Here's how the part is built. I have some questions about the finished solid (model axes, mm). A direction names the side the tool comes from. Give positions to 0.01 mm unless a question says otherwise; leave off trailing zeros. Write each loop counter-clockwise with the first axis right and the second up, starting at its lowest first coordinate (ties: lowest second). Pieces come first, ordered by that corner, then holes. Notation, with made-up numbers: (-24.75, 84.25) -> (-9.75, 84.25) arc R23 cw to (-9.75, 98.25) -> close; hole circle Ø5 at (28, 51). An arc over 180 degrees is marked (long way). Put each result on its own line as item: value. Start each with the question number.
from build123d import *

# Parameters (mm, degrees)
BOSS_EXTRUDE1_DEPTH = 20
SKETCH2_R           = 35
SKETCH2_R_2         = 20
BOSS_EXTRUDE2_DEPTH = 30
FILLET1_R           = 2
FILLET2_R           = 2


with BuildPart() as part:
    # Sketch1 → Revolve-Thin1 (revolve)
    with BuildSketch(Plane.XY, mode=Mode.PRIVATE) as revolve_thin1_sk:
        with BuildLine():
            Line((56.568542495, 20), (80, 20))
            ThreePointArc((80, 20), (81.025996139, 15.83772234), (84.898979486, 14))
            Line((84.898979486, 14), (150, 14))
            Line((150, 14), (150, 0))
            Line((150, 0), (140, 0))
            Line((140, 0), (140, 4))
            Line((140, 4), (84.898979486, 4))
            ThreePointArc((84.898979486, 4), (78.190775553, 5.583592135), (72.898979486, 10))
            Line((72.898979486, 10), (56.568542495, 10))
            Line((56.568542495, 10), (56.568542495, 20))
        make_face()
    revolve(revolve_thin1_sk.sketch.rotate(Axis((-93.302775415, 0, 0), (1, 0, 0)), 90), axis=Axis((-93.302775415, 0, 0), (1, 0, 0)))

    # Sketch1<4> → Boss-Extrude1 (add, symmetric)
    with BuildSketch(Plane.XY):
        with BuildLine():
            Line((0, 60), (-21.3, 60))
            Line((-21.3, 60), (-21.3, 40))
            Line((-21.3, 40), (0, 40))
            ThreePointArc((0, 40), (40, 0), (0, -40))
            Line((0, -40), (-21.3, -40))
            Line((-21.3, -40), (-21.3, -60))
            Line((-21.3, -60), (0, -60))
            ThreePointArc((0, -60), (60, 0), (0, 60))
        make_face()
    extrude(amount=BOSS_EXTRUDE1_DEPTH, both=True)

    # Sketch2 → Boss-Extrude2 (add)
    with BuildSketch(Plane(origin=(0, 40, 0), x_dir=(1, 0, 0), z_dir=(0, 1, 0))):
        with Locations(Location((-50, 0, 0), (0, 0, 34.849904579))):
            Circle(SKETCH2_R)
        with Locations(Location((-50, 0, 0), (0, 0, 270))):
            Circle(SKETCH2_R_2, mode=Mode.SUBTRACT)
    boss_extrude2 = extrude(amount=BOSS_EXTRUDE2_DEPTH)

    # Fillet1
    # the kernel refuses this fillet: 2 mm, written as the material it adds along each edge
    with BuildSketch(Plane(origin=(-50, 60, 0), x_dir=(0.7309132797972386, 0, -0.682470349111259), z_dir=(-0.682470349111259, 0, -0.7309132797972386))) as fillet1_piece_1_section:
        with BuildLine():
            CenterArc((35 + FILLET1_R, -FILLET1_R), FILLET1_R, 90, 90)
            Line((35, -FILLET1_R), (35, 0))
            Line((35, 0), (35 + FILLET1_R, 0))
        make_face()
    fillet1_piece_1 = revolve(axis=Axis((-50, 60, 0), (0, -1, 0)), revolution_arc=86.073975491, mode=Mode.PRIVATE)
    fillet1_piece_1 = split(fillet1_piece_1, bisect_by=Plane(origin=(-14.43905365, 60.56094635, -20), z_dir=(0, 0, 1)), keep=Keep.TOP, mode=Mode.PRIVATE)
    fillet1_piece_1 = split(fillet1_piece_1, bisect_by=Plane(origin=(-14.43905365, 60.56094635, 20), z_dir=(0, 0, -1)), keep=Keep.TOP, mode=Mode.PRIVATE)
    add(fillet1_piece_1)

    # Mirror3: Boss-Extrude2 across plane
    add(boss_extrude2.mirror(Plane.ZX))

    # Fillet2
    # the kernel refuses this fillet: 2 mm, written as the material it adds along each edge
    with BuildSketch(Plane(origin=(-50, -60, 0), x_dir=(0.7309132797966846, 0, 0.6824703491118522), z_dir=(-0.6824703491118522, 0, 0.7309132797966846))) as fillet2_piece_1_section:
        with BuildLine():
            CenterArc((35 + FILLET2_R, -FILLET2_R), FILLET2_R, 90, 90)
            Line((35, -FILLET2_R), (35, 0))
            Line((35, 0), (35 + FILLET2_R, 0))
        make_face()
    fillet2_piece_1 = revolve(axis=Axis((-50, -60, 0), (0, 1, 0)), revolution_arc=86.073975491, mode=Mode.PRIVATE)
    fillet2_piece_1 = split(fillet2_piece_1, bisect_by=Plane(origin=(-14.439053646, -60.560946354, -20), z_dir=(0, 0, 1)), keep=Keep.TOP, mode=Mode.PRIVATE)
    fillet2_piece_1 = split(fillet2_piece_1, bisect_by=Plane(origin=(-14.439053646, -60.560946354, 20), z_dir=(0, 0, -1)), keep=Keep.TOP, mode=Mode.PRIVATE)
    add(fillet2_piece_1)


solid = part.part
1) I'm going to push flat-ended pins straight in: pin 1 Ø5 at (x, z) = (28, -14) entering from +Y; pin 2 Ø9 at (y, z) = (0, 0) entering from -X; pin 3 Ø1 at (y, z) = (37.5, 3.5) entering from +X. Where does each tip first touch, or does it pass through?
2) I want a section at B-B, the plane z = 0. State how many separate pieces and enclosed holes the cut face has, and give its area (3 significant figures).
3) I want a section at A-A, the plane x = -50. Write out the boundary of the cut face in (y, z), and give its area (3 significant figures).
4) I want a section at D-D, the plane z = 30. Write out the boundary of the cut face in (x, y), and give its area (3 significant figures).
5) Thinking about a two-plate mould opening in Z: for faces 1 (the cylindrical face through (-84.687, 54.79, -4.671)), 2 (the flat face through (150, 0, 0)), 3 (the cylindrical face through (-30.17, 54.79, -2.6)), which applies, released by +Z, released by -Z, zero draft, split by the parting line, or undercut?
6) I need wall thicknesses on probe 1 along Y at (x, z) = (106, 0); probe 2 along Y at (x, z) = (62, 0); probe 3 along Z at (x, y) = (17.5, -56.5). Which ranges of each line are inside material? Lowest first, please.
7) I want a section at C-C, the plane x = 21. Write out the boundary of the cut face in (y, z), and give its area (3 significant figures).
8) Which directions (+Z, -Z, +X, -X, +Y, -Y) give clear straight access to the entire face, cutting with the end or side of a thin tool? Please do faces 4 (the cylindrical face through (117.9, 12.4, 6.5)), 5 (the cylindrical face through (60, 0, 0)), 6 (the flat face through (-28, -40, 1)).
Established:
1. pin 1: stops at y = 54.31
1. pin 2: stops at x = 39.75
1. pin 3: stops at x = 47.23
2. separate pieces: 3
2. enclosed holes: 1
2. area: 7,510 mm2
3. outline: (-70, -35) -> (-40, -35) -> (-40, -20) -> (-70, -20) -> close; (-70, 20) -> (-40, 20) -> (-40, 35) -> (-70, 35) -> close; (40, -35) -> (70, -35) -> (70, -20) -> (40, -20) -> close; (40, 20) -> (70, 20) -> (70, 35) -> (40, 35) -> close
3. area: 1,800 mm2
4. outline: (-68.03, -70) -> (-31.97, -70) -> (-31.97, -40) -> (-68.03, -40) -> close; (-68.03, 40) -> (-31.97, 40) -> (-31.97, 70) -> (-68.03, 70) -> close
4. area: 2,160 mm2
5. face 1: split by the parting line
5. face 2: zero draft
5. face 3: undercut
6. probe 1: y = -14 to -4, 4 to 14
6. probe 2: y = -20 to -10, 10 to 20
6. probe 3: z = -20 to 20
7. outline: (-56.2, -20) -> (-34.04, -20) -> (-34.04, 20) -> (-56.2, 20) -> close; (34.04, -20) -> (56.2, -20) -> (56.2, 20) -> (34.04, 20) -> close
7. area: 1,770 mm2
8. face 4: +X
8. face 5: none
8. face 6: +Z, -Z, -X
